The listing builds one solid part. Answer for the finished solid, in the listing's coordinates (mm). Face numbers are marked on the shaded views. A direction names the side the tool comes from. Give positions to 0.01 mm unless a question says otherwise; leave off trailing zeros. Write each loop counter-clockwise with the first axis right and the second up, starting at its lowest first coordinate (ties: lowest second). Pieces come first, ordered by that corner, then holes.
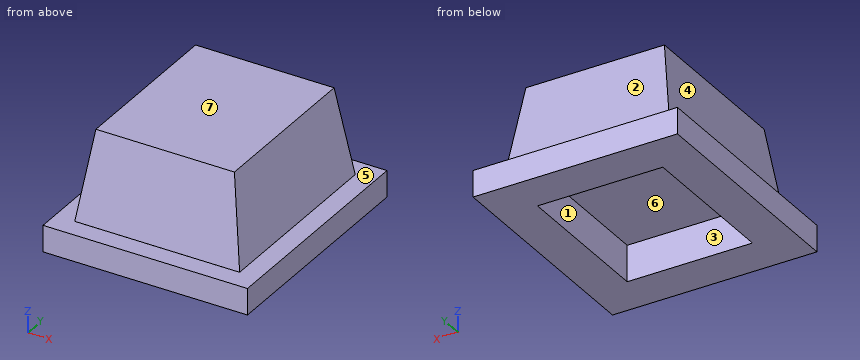
Autodesk Fusion 360 part; units mm, degrees
sketch "Sketch1" plane through (0, 0, 0) normal (0, 0, 1) x (1, 0, 0)
  line L0 (0, 0) -> (5, 0)
  line L1 (5, 0) -> (5, 5.8)
  line L2 (5, 5.8) -> (0, 5.8)
  line L3 (0, 5.8) -> (0, 0)
  dimension "d1" = 5
  dimension "d2" = 5.8
extrude "Extrude1" add sketch "Sketch1" along normal blind 3.5
sketch "Sketch2" plane through (0, 0, 0) normal (0, 0, -1) x (-1, 0, 0)
  line L0 (0, 0) -> (0, 5.8)
  line L1 (0, 5.8) -> (-5, 5.8)
  line L2 (-5, 5.8) -> (-5, 0)
  line L3 (-5, 0) -> (0, 0)
  line L4 (-4.4, 5.15) -> (-0.6, 5.15)
  line L5 (-0.6, 5.15) -> (-0.6, 0.65)
  line L6 (-0.6, 0.65) -> (-4.4, 0.65)
  line L7 (-4.4, 0.65) -> (-4.4, 5.15)
  dimension "d5" = 3.8
  dimension "d6" = 4.5
  dimension "d7" = 0.6
  dimension "d8" = 0.65
extrude "Extrude2" cut sketch "Sketch2" against normal blind 1.1 contours L4 L5 L6 L7
sketch "Sketch3" plane through (0, 0, 0) normal (0, 0, -1) x (-1, 0, 0)
  line L0 (-0.6, 5.15) -> (-0.6, 0.65)
  line L1 (-0.6, 0.65) -> (-4.4, 0.65)
  line L2 (-4.4, 0.65) -> (-4.4, 5.15)
  line L3 (-4.4, 5.15) -> (-0.6, 5.15)
  line L4 (0, 0) -> (0, 5.8)
  line L5 (0, 5.8) -> (-5, 5.8)
  line L6 (-5, 5.8) -> (-5, 0)
  line L7 (-5, 0) -> (0, 0)
  line L8 (-5.6, 6.4) -> (0.6, 6.4)
  line L9 (0.6, 6.4) -> (0.6, -0.6)
  line L10 (0.6, -0.6) -> (-5.6, -0.6)
  line L11 (-5.6, -0.6) -> (-5.6, 6.4)
  dimension "d11" = 0.6
  dimension "d12" = 0.6
  dimension "d13" = 0.6
  dimension "d14" = 0.6
extrude "Extrude3" add sketch "Sketch3" against normal blind 0.8 contours L8 L9 L10 L11
chamfer "Chamfer1" distance 0.4 distance2 2.7 4 edges at (5, 2.9, 3.5) (2.5, 5.8, 3.5) (0, 2.9, 3.5) (2.5, 0, 3.5) measured on face at (1.6667, 3.8667, 3.5) measured on face at (1.6667, 3.8667, 3.5) measured on face at (1.6667, 3.8667, 3.5) measured on face at (1.6667, 3.8667, 3.5)
Item 1: A cutting plane is placed at A-A, the plane z = 0.6. Give the vertices of the cut face in (x, y).
Conclusion:
outline: (-0.6, -0.6) - (5.6, -0.6) - (5.6, 6.4) - (-0.6, 6.4) - close; hole (0.6, 0.65) - (4.4, 0.65) - (4.4, 5.15) - (0.6, 5.15) - close
Item 2: Each of these flat-tipped pins is pushed along its axis until it touches: P1, Ø1, axis at x = 4.5, z = 1, coming from the +Y side; P2, Ø1.5, axis at x = 1.5, z = 2.5, coming from the -Y side. Where does it stop, or does it pass through?
Conclusion:
P1: stops at y = 6.4
P2: stops at y = 0.14
Item 3: Consider probe 1 along Y at (x, z) = (4.25, 0.35); probe 2 along X at (y, z) = (4.75, 0.65); probe 3 along Z at (x, y) = (3, 4). Determine where each line is inside the solid, lowest interval first.
Conclusion:
probe 1: y = -0.6 to 0.65, 5.15 to 6.4
probe 2: x = -0.6 to 0.6, 4.4 to 5.6
probe 3: z = 1.1 to 3.5
Item 4: Which of the six approach directions +Z, -Z, +X, -X, +Y, -Y give full straight-line access (tool end or side, diameter ignored) to the marked faces 5, 6 and 7?
Conclusion:
face 5: +Z
face 6: -Z
face 7: +Z, +X, -X, +Y, -Y
Item 5: Determine the mould class of the marked faces 1, 2, 3 and 4 for opening direction X: pulls with the +X half, pulls with the -X half, needs draft (parallel to the pull), parting line crosses it, or undercut.
Conclusion:
face 1: undercut
face 2: needs draft
face 3: undercut
face 4: pulls with the -X half
